from build123d import *

# Parameters (mm, degrees)
SKETCH1_R           = 15
SKETCH1_R_2         = 6
BOSS_EXTRUDE1_DEPTH = 5


with BuildPart() as part:
    # Sketch1 → Boss-Extrude1 (new body)
    with BuildSketch(Plane(origin=(0, 0, 0), x_dir=(1, 0, 0), z_dir=(0, 1, 0))):
        with BuildLine():
            Line((114.772255751, 30), (150, 30))
            ThreePointArc((150, 30), (153.535533906, 28.535533906), (155, 25))
            Line((155, 25), (155, 0))
            Line((155, 0), (0, 0))
            Line((0, 0), (0, 105))
            ThreePointArc((0, 105), (1.464466094, 108.535533906), (5, 110))
            Line((5, 110), (55, 110))
            ThreePointArc((55, 110), (58.535533906, 108.535533906), (60, 105))
            Line((60, 105), (60, 84.772255751))
            ThreePointArc((60, 84.772255751), (61.307255271, 81.401256438), (64.545454545, 79.792959773))
            ThreePointArc((64.545454545, 79.792959773), (95.355339059, 65.355339059), (109.792959773, 34.545454545))
            ThreePointArc((109.792959773, 34.545454545), (111.401256438, 31.307255271), (114.772255751, 30))
        make_face()
        with Locations(Location((30, 90, 0), (0, 0, 270))):
            Circle(SKETCH1_R, mode=Mode.SUBTRACT)
        with Locations(Location((20, 15, 0), (0, 0, 270))):
            Circle(SKETCH1_R_2, mode=Mode.SUBTRACT)
        with Locations(Location((40, 15, 0), (0, 0, 270))):
            Circle(SKETCH1_R_2, mode=Mode.SUBTRACT)
        with Locations(Location((60, 15, 0), (0, 0, 270))):
            Circle(SKETCH1_R_2, mode=Mode.SUBTRACT)
        with Locations(Location((80, 15, 0), (0, 0, 270))):
            Circle(SKETCH1_R_2, mode=Mode.SUBTRACT)
        with Locations(Location((100, 15, 0), (0, 0, 270))):
            Circle(SKETCH1_R_2, mode=Mode.SUBTRACT)
        with Locations(Location((120, 15, 0), (0, 0, 270))):
            Circle(SKETCH1_R_2, mode=Mode.SUBTRACT)
        with Locations(Location((140, 15, 0), (0, 0, 270))):
            Circle(SKETCH1_R_2, mode=Mode.SUBTRACT)
        with BuildLine():
            Line((20, 55), (20, 35))
            ThreePointArc((20, 35), (21.464466094, 31.464466094), (25, 30))
            Line((25, 30), (84.494897428, 30))
            ThreePointArc((84.494897428, 30), (88.367880774, 31.83772234), (89.393876913, 36))
            ThreePointArc((89.393876913, 36), (78.973665961, 53.237900077), (60, 60))
            Line((60, 60), (25, 60))
            ThreePointArc((25, 60), (21.464466094, 58.535533906), (20, 55))
        make_face(mode=Mode.SUBTRACT)
    extrude(amount=BOSS_EXTRUDE1_DEPTH)


solid = part.part
Verification items for the finished model (mm, model axes). A direction names the side the tool comes from. Round coordinates to 2 decimals unless told otherwise and drop trailing zeros. Order: outer loops, then holes, each group sorted by start corner. A loop starts at its lowest first (then second) coordinate and runs counter-clockwise, first axis right, second up.
1. Go/stop test with flat-tipped pins: P1, Ø3, axis at y = 1, z = -97.5, coming from the +X side; P2, Ø1, axis at x = 69, y = 1.5, coming from the -Z side; P3, Ø1.5, axis at y = 3.5, z = -46, coming from the +X side; P4, Ø7, axis at x = 100, z = -15, coming from the +Y side. Record where each tip stops, or that it passes through.
Final values:
P1: stops at x = 60
P2: stops at z = -79.27
P3: stops at x = 107.62
P4: passes through
2. Access from +Z, -Z, +X, -X, +Y, -Y to the whole of each face (thin tool, end or side, straight path). Record for faces 1 (the cylindrical face through (1, 2, -108)), 2 (the flat face through (60, 2, -95)), 3 (the cylindrical face through (88.33, 2.46, -31.79)).
Final values:
face 1: -Z, -X, +Y, -Y
face 2: -Z, +X, +Y, -Y
face 3: +Y, -Y
3. Release check for a two-part mould opening along X. For faces 4 (the flat face through (155, 2, -13)), 5 (the flat face through (54, 2, -30)), 6 (the flat face through (79, 5, -56)) record: +X half, -X half, draft (parallel to the pull), parting line (faces both ways), or undercut.
Final values:
face 4: +X half
face 5: undercut
face 6: draft
4. Section check B-B on z = -15. State how many separate pieces and enclosed holes the cut face has, then the cut area to 3 significant figures.
Final values:
separate pieces: 8
enclosed holes: 0
area: 355 mm2
5. Section check A-A on x = 100. Record the cut outline in (y, z).
Final values:
outline: (0, -60) - (5, -60) - (5, -21) - (0, -21) - close; (0, -9) - (5, -9) - (5, 0) - (0, 0) - close
6. Thickness scan on L1, parallel to Z at x = 20.5, y = 1.3; L2, parallel to Z at x = 28.5, y = 3.95; L3, parallel to Z at x = 51, y = 1.05. Record the ranges inside material, lowest first.
Final values:
L1: z = -110 to -101.61, -78.39 to -57.18, -32.82 to -20.98, -9.02 to 0
L2: z = -110 to -104.92, -75.08 to -60, -30 to 0
L3: z = -110 to -60, -30 to 0
7. Section check D-D on x = 40. Record the cut outline in (y, z).
Final values:
outline: (0, -110) - (5, -110) - (5, -101.18) - (0, -101.18) - close; (0, -78.82) - (5, -78.82) - (5, -60) - (0, -60) - close; (0, -30) - (5, -30) - (5, -21) - (0, -21) - close; (0, -9) - (5, -9) - (5, 0) - (0, 0) - close
